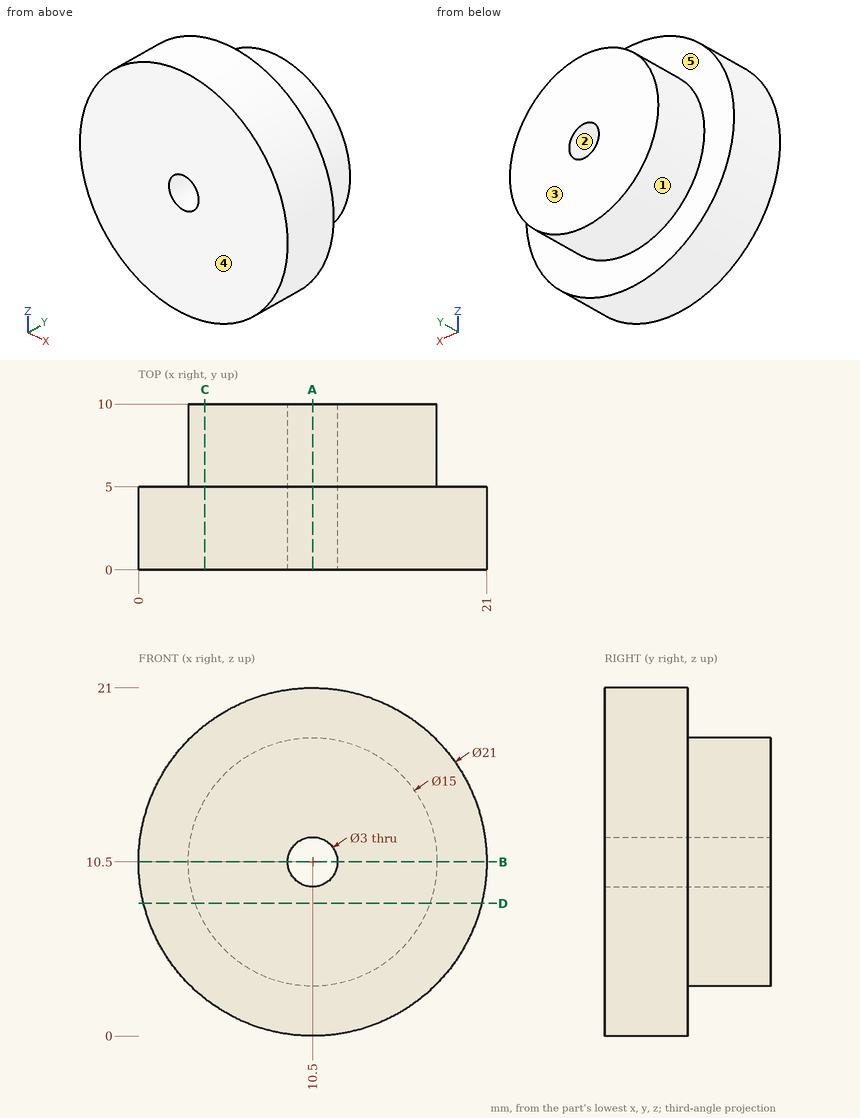
Part print with two shaded views. Sizes in mm from the minimum x, y, z corner. A direction names the side the tool comes from. Give positions to 0.01 mm unless a question says otherwise; leave off trailing zeros. Order: outer loops, then holes, each group sorted by start corner. A loop starts at its lowest first (then second) coordinate and runs counter-clockwise, first axis right, second up.
(1) Flat gauge pins, fed straight in: pin 1 (1 mm diameter, centred on y = 8, z = 5, fed in from -X); pin 2 (1.5 mm diameter, centred on y = 1.5, z = 8, fed in from +X); pin 3 (1 mm diameter, centred on y = 6.5, z = 14.5, fed in from +X). Where does each tip first touch, or does it go through?
(2) Saw through at B-B, the plane z = 10.5. Give the cut face in (x, y).
(3) Mould opens along X. For the marked faces 1, 2 and 3 say: released by +X, released by -X, zero draft, split by the parting line, or undercut.
(4) Saw through at D-D, the plane z = 8. Give the cut face in (x, y), then the cut area to 3 significant figures.
(5) Saw through at C-C, the plane x = 4. Give the cut face in (y, z).
(6) Saw through at A-A, the plane x = 10.5. Give the cut face in (y, z), then the cut area to 3 significant figures.
(7) Tool access for the marked faces 4 and 5: list every direction of +Z, -Z, +X, -X, +Y, -Y with a clear straight run to the whole face (end or side of a thin tool).
(8) Drill centre lines: L1, parallel to X at y = 6, z = 10.5; L2, parallel to Y at x = 15.75, z = 2.5. Where is each one in solid material? Low to high.
Results found:
1. pin 1: stops at x = 4.91
1. pin 2: stops at x = 20.85
1. pin 3: stops at x = 17.13
2. outline: (0, 0) - (9, 0) - (9, 10) - (3, 10) - (3, 5) - (0, 5) - close; (12, 0) - (21, 0) - (21, 5) - (18, 5) - (18, 10) - (12, 10) - close
3. face 1: split by the parting line
3. face 2: undercut
3. face 3: zero draft
4. outline: (0.3, 0) - (20.7, 0) - (20.7, 5) - (17.57, 5) - (17.57, 10) - (3.43, 10) - (3.43, 5) - (0.3, 5) - close
4. area: 173 mm2
5. outline: (0, 2.25) - (5, 2.25) - (5, 6.76) - (10, 6.76) - (10, 14.24) - (5, 14.24) - (5, 18.75) - (0, 18.75) - close
6. outline: (0, 0) - (5, 0) - (5, 3) - (10, 3) - (10, 9) - (0, 9) - close; (0, 12) - (10, 12) - (10, 18) - (5, 18) - (5, 21) - (0, 21) - close
6. area: 150 mm2
7. face 4: +Z, -Z, +X, -X, -Y
7. face 5: +Y
8. L1: x = 3 to 9, 12 to 18
8. L2: y = 0 to 5
